Input: part model. Units: mm. Frame: model coordinates. Face numbers are marked on the shaded views. A direction names the side the tool comes from. Round coordinates to 2 decimals unless told otherwise and drop trailing zeros. Loops run counter-clockwise (first coordinate to the right, second up) from the corner with the lowest first, then second, coordinate; pieces in that order, holes last. Notation, with made-up numbers: (34.25, 51) -> (42.25, 51) arc R14 cw to (42.25, 77) -> close; hole circle Ø3 at (-37.5, -26.75). An arc over 180 degrees is marked (long way). Answer as a JSON object with one key per item and string values.
```python
from build123d import *

# Parameters (mm, degrees)
F0_W     = 80
F0_H     = 80
F1_DEPTH = 45
F3_DEPTH = 25
F4_DEPTH = 25
F5_W     = 35
F5_H     = 80
F5_W_2   = 25
F6_DEPTH = 5


with BuildPart() as f1:
    # F0 (on Front) → F1 (new body)
    with BuildSketch(Plane.XZ):
        Rectangle(F0_W, F0_H)
    extrude(amount=F1_DEPTH)

    # F2 (on face) → F3 (join)
    with BuildSketch(Plane.XZ.offset(45)):
        Polygon((30, -25), (30, -40), (40, -40), (40, 15), (-10, 15), align=None)
    extrude(amount=F3_DEPTH)

    # F2 (on face) → F4 (join)
    with BuildSketch(Plane.XZ.offset(45)):
        Polygon((-20, 15), (-10, 15), (40, 15), (40, 40), (-20, 40), align=None)
    extrude(amount=F4_DEPTH)

    # F5 (on face) → F6 (cut)
    with BuildSketch(Plane(origin=(0, 0, 0), x_dir=(-1, 0, 0), z_dir=(0, 1, 0))):
        with Locations((-22.5, 0)):
            Rectangle(F5_W, F5_H)
        with Locations((27.5, 0)):
            Rectangle(F5_W_2, F5_H)
    extrude(amount=-F6_DEPTH, mode=Mode.SUBTRACT)


solid = f1.part
```
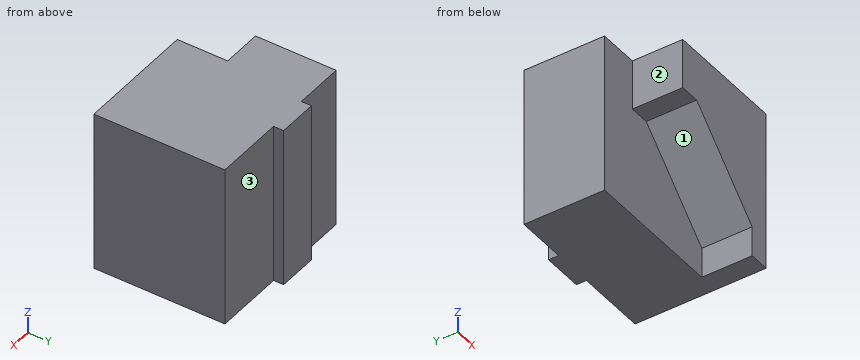
1) Section A-A, the plane z = -33. Output: boundary loops of the cut face in (x, y).
Output:
{"outline": "(-40, -45) -> (30, -45) -> (30, -70) -> (40, -70) -> (40, -5) -> (5, -5) -> (5, 0) -> (-15, 0) -> (-15, -5) -> (-40, -5) -> close"}
2) Ray query, probe 1 along Y at (x, z) = (-35, 7); probe 2 along Y at (x, z) = (19, -7); probe 3 along X at (y, z) = (-3.5, 15). Return the intervals inside material, ascending.
Output:
{"probe 1": "y = -45 to -5", "probe 2": "y = -70 to -5", "probe 3": "x = -15 to 5"}
3) Reachability of the marked faces 1, 2 and 3 from +Z, -Z, +X, -X, +Y, -Y: full face, straight path, thin tool, end or side. Return the list, or none.
Output:
{"face 1": "-Z, -X, -Y", "face 2": "+Z, -Z, -X, -Y", "face 3": "+Z, -Z, +X, +Y"}
4) Contact query for flat-ended pins moving along their axis: P1, Ø7.5, axis at y = -57, z = 30, coming from the -X side; P2, Ø20, axis at x = -26.5, z = -3.5, coming from the +Y side; P3, Ø1.5, axis at y = -3, z = 14.5, coming from the -X side. Output: stop coordinate, or through.
Output:
{"P1": "stops at x = -20", "P2": "stops at y = -5", "P3": "stops at x = -15"}
5) Section D-D, the plane z = 10.5. Output: boundary loops of the cut face in (x, y), plus the area to 3 significant figures.
Output:
{"outline": "(-40, -45) -> (-5.5, -45) -> (-5.5, -70) -> (40, -70) -> (40, -5) -> (5, -5) -> (5, 0) -> (-15, 0) -> (-15, -5) -> (-40, -5) -> close", "area": "4,440 mm^2"}
6) Section B-B, the plane y = -53. Output: boundary loops of the cut face in (x, z), plus the area to 3 significant figures.
Output:
{"outline": "(-20, 15) -> (-10, 15) -> (30, -25) -> (30, -40) -> (40, -40) -> (40, 40) -> (-20, 40) -> close", "area": "2,850 mm^2"}
7) Section C-C, the plane x = 23. Output: boundary loops of the cut face in (y, z).
Output:
{"outline": "(-70, -18) -> (-45, -18) -> (-45, -40) -> (-5, -40) -> (-5, 40) -> (-70, 40) -> close"}
